from build123d import *

# Parameters (mm, degrees)
SKETCH1_W           = 12.7
SKETCH1_H           = 6.35
SKETCH1_R           = 1.9939
SKETCH1_R_2         = 0.9652
BOSS_EXTRUDE1_DEPTH = 7.0612
SKETCH1_3_R         = 1.9939
SKETCH1_3_R_2       = 0.9652
CUT_EXTRUDE1_DEPTH  = 3.556


with BuildPart() as part:
    # Sketch1 → Boss-Extrude1 (new body)
    # profile 1 of 3: a face of its own
    with BuildSketch(Plane.XY):
        Rectangle(SKETCH1_W, SKETCH1_H)
        with Locations((-3.3782, 0)):
            Circle(SKETCH1_R, mode=Mode.SUBTRACT)
        with Locations((3.3782, 0)):
            Circle(SKETCH1_R, mode=Mode.SUBTRACT)
    # profile 2 of 3: a face of its own
    with BuildSketch(Plane.XY):
        with Locations((-3.3782, 0)):
            Circle(SKETCH1_R)
        with Locations((-3.3782, 0)):
            Circle(SKETCH1_R_2, mode=Mode.SUBTRACT)
    # profile 3 of 3: a face of its own
    with BuildSketch(Plane.XY):
        with Locations((3.3782, 0)):
            Circle(SKETCH1_R)
        with Locations((3.3782, 0)):
            Circle(SKETCH1_R_2, mode=Mode.SUBTRACT)
    extrude(amount=BOSS_EXTRUDE1_DEPTH)

    # Sketch1_3 → Cut-Extrude1 (cut)
    # profile 1 of 2: a face of its own
    with BuildSketch(Plane.XY):
        with Locations((3.3782, 0)):
            Circle(SKETCH1_3_R)
        with Locations((3.3782, 0)):
            Circle(SKETCH1_3_R_2, mode=Mode.SUBTRACT)
    # profile 2 of 2: a face of its own
    with BuildSketch(Plane.XY):
        with Locations((-3.3782, 0)):
            Circle(SKETCH1_3_R)
        with Locations((-3.3782, 0)):
            Circle(SKETCH1_3_R_2, mode=Mode.SUBTRACT)
    extrude(amount=CUT_EXTRUDE1_DEPTH, mode=Mode.SUBTRACT)


solid = part.part
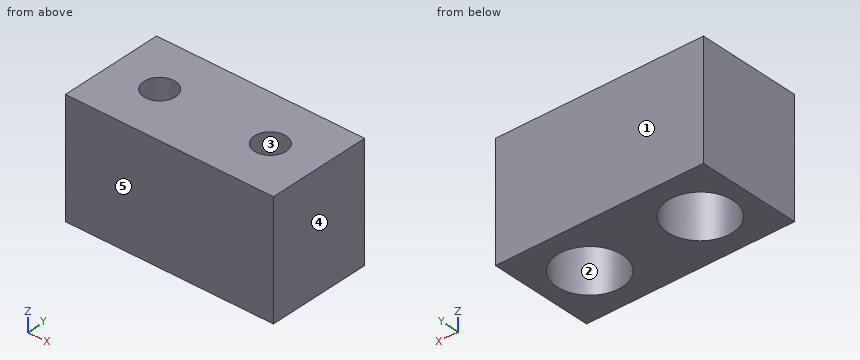
Design review of the part built by this model. Coordinates are the model's own, in mm. Face numbers are marked on the shaded views. A direction names the side the tool comes from. Give positions to 0.01 mm unless a question says otherwise; leave off trailing zeros. Loops run counter-clockwise (first coordinate to the right, second up) from the corner with the lowest first, then second, coordinate; pieces in that order, holes last. Notation, with made-up numbers: M -40,66 L -18,66 A23 ccw -18,80 Z; hole C 74,2.25 d8. An arc over 180 degrees is marked long. Answer as a JSON object with one key per item and string values.
Item 1: We need section B-B (z = 5.75). State the section outline as (x, y) points (3 decimals).
Output values:
{"outline": "M -6.35,-3.175 L 6.35,-3.175 L 6.35,3.175 L -6.35,3.175 Z; hole C -3.378,0 d1.93; hole C 3.378,0 d1.93"}
Item 2: For P1, Ø3.5, axis at x = -3.38, y = 0, coming from the +Z side; P2, Ø1.2, axis at x = 3.5, y = 0.5, coming from the -Z side; P3, Ø1.7, axis at x = 3.38, y = 0, coming from the -Z side, all flat-tipped, find the tip position at first contact; note any pin that passes through.
Output values:
{"P1": "stops at z = 7.06", "P2": "stops at z = 3.56", "P3": "passes through"}
Item 3: Wall thickness on line 1 along Y through (x, z) = (-3.5, 0.5) (3 decimals); line 2 along X through (y, z) = (1.5, 1); line 3 along Z through (x, y) = (2.5, -0.5): over which ranges is each line inside the solid? List them lowest first.
Output values:
{"line 1": "y = -3.175 to -1.99, 1.99 to 3.175", "line 2": "x = -6.35 to -4.69, -2.06 to 2.06, 4.69 to 6.35", "line 3": "z = 3.56 to 7.06"}
Item 4: We need section A-A (y = 0). State the section outline as (x, z) points.
Output values:
{"outline": "M -6.35,0 L -5.37,0 L -5.37,3.56 L -4.34,3.56 L -4.34,7.06 L -6.35,7.06 Z; M -2.41,3.56 L -1.38,3.56 L -1.38,0 L 1.38,0 L 1.38,3.56 L 2.41,3.56 L 2.41,7.06 L -2.41,7.06 Z; M 4.34,3.56 L 5.37,3.56 L 5.37,0 L 6.35,0 L 6.35,7.06 L 4.34,7.06 Z"}
Item 5: We need section C-C (x = 5). State the section outline as (y, z) points (3 decimals), and give its area (3 significant figures).
Output values:
{"outline": "M -3.175,0 L -1.16,0 L -1.16,3.556 L 1.16,3.556 L 1.16,0 L 3.175,0 L 3.175,7.061 L -3.175,7.061 Z", "area": "36.6 mm2"}
Item 6: Machinability: for the marked faces 1 and 2, which of the approach directions +Z, -Z, +X, -X, +Y, -Y give a long, thin tool a straight path to every point of the face, cutting with its end or side? Answer none if there is none.
Output values:
{"face 1": "+Z, -Z, +X, -X, +Y", "face 2": "-Z"}
Item 7: Mouldability with a two-part tool opening along Y and no side actions: class the marked faces 3, 4 and 5 as pulls with the +Y half, pulls with the -Y half, needs draft (parallel to the pull), parting line crosses it, or undercut.
Output values:
{"face 3": "undercut", "face 4": "needs draft", "face 5": "pulls with the -Y half"}
Item 8: We need section D-D (z = 3.25). State the section outline as (x, y) points (3 decimals).
Output values:
{"outline": "M -6.35,-3.175 L 6.35,-3.175 L 6.35,3.175 L -6.35,3.175 Z; hole C -3.378,0 d3.988; hole C 3.378,0 d3.988"}
